For this review, take the finished solid that the model builds, in its own axes (mm). Face numbers are marked on the shaded views. A direction names the side the tool comes from. Give positions to 0.01 mm unless a question says otherwise; leave off trailing zeros. Loops run counter-clockwise (first coordinate to the right, second up) from the corner with the lowest first, then second, coordinate; pieces in that order, holes last. Notation, with made-up numbers: (26.25, -29) - (38.25, -29) arc R25 ccw to (38.25, -15) - close; hole circle Ø11 at (49.5, 51.25). An arc over 180 degrees is marked (long way). Answer in a Markdown table with one row per item.
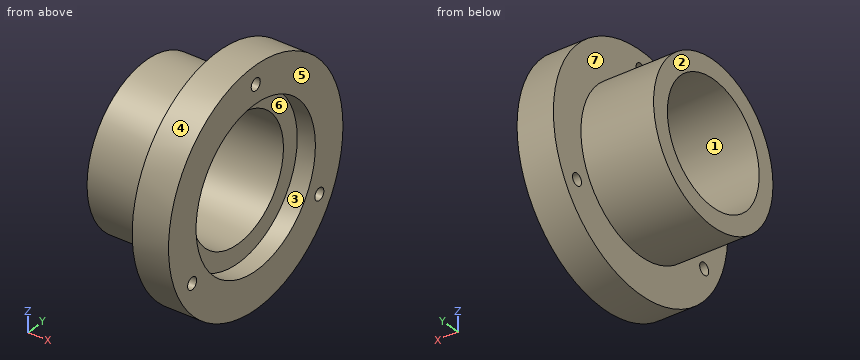
```python
from build123d import *

# Parameters (mm, degrees)
F0_R        = 24.13
F1_DEPTH    = 22.86
F2_R        = 16.51
F3_DEPTH    = 3.81
F4_R        = 12.7
F5_DEPTH    = 19.05
F6_R        = 24.13
F6_R_2      = 16.51
F7_DEPTH    = 15.24
F8_R        = 1.25
F7_FACE_R   = 24.13
F7_FACE_R_2 = 16.51
F9_DEPTH    = 25.4


with BuildPart() as f1:
    # F0 (on Right) → F1 (new body)
    with BuildSketch(Plane.YZ):
        Circle(F0_R)
    extrude(amount=F1_DEPTH)

    # F2 (on face) → F3 (cut)
    with BuildSketch(Plane.YZ.offset(22.86)):
        Circle(F2_R)
    extrude(amount=-F3_DEPTH, mode=Mode.SUBTRACT)

    # F4 (on face) → F5 (cut, through all)
    with BuildSketch(Plane.YZ.offset(19.05)):
        Circle(F4_R)
    extrude(amount=-F5_DEPTH, mode=Mode.SUBTRACT)

    # F6 (on face) → F7 (cut)
    with BuildSketch(Plane(origin=(0, 0, 0), x_dir=(0, -1, 0), z_dir=(-1, 0, 0))):
        Circle(F6_R)
        Circle(F6_R_2, mode=Mode.SUBTRACT)
    extrude(amount=-F7_DEPTH, mode=Mode.SUBTRACT)

    # F8 (on face) + F7_face (on face) → F9 (cut)
    with BuildSketch(Plane.YZ.offset(22.86)):
        with Locations((0, 20.32)):
            Circle(F8_R)
        with Locations((-17.5976362049, -10.16)):
            Circle(F8_R)
        with Locations((17.5976362049, -10.16)):
            Circle(F8_R)
    with BuildSketch(Plane(origin=(15.24, 0, 0), x_dir=(0, -1, 0), z_dir=(-1, 0, 0))):
        Circle(F7_FACE_R)
        Circle(F7_FACE_R_2, mode=Mode.SUBTRACT)
    extrude(amount=-F9_DEPTH, dir=(1, 0, 0), mode=Mode.SUBTRACT)


solid = f1.part
```
1. Clearance check with flat-ended pins moving along their axes: pin 1 (3 mm diameter, centred on y = 17.6, z = -10.16, fed in from -X); pin 2 (2 mm diameter, centred on x = 6.5, y = -11, fed in from +Z); pin 3 (16.5 mm diameter, centred on y = 1.5, z = -1.5, fed in from +X); pin 4 (2 mm diameter, centred on x = 16, y = -15.5, fed in from -Z). State where each tip first meets the part, or that it passes through.
Values:
| item | result |
|---|---|
| pin 1 | stops at x = 15.24 |
| pin 2 | stops at z = 13.14 |
| pin 3 | passes through |
| pin 4 | stops at z = -19.29 |
2. For the marked faces 5, 6 and 7, list the 3-axis set-ups (+Z, -Z, +X, -X, +Y, -Y) from which the entire face can be reached by the end or side of a thin tool; tool diameter is ignored.
Values:
| item | result |
|---|---|
| face 5 | +Z, -Z, +X, +Y, -Y |
| face 6 | +X |
| face 7 | -X |
3. We need section D-D, the plane z = -10.16. Give the boundary of the cut face in (x, y), and give its area (3 significant figures).
Values:
| item | result |
|---|---|
| outline | (0, -13.01) - (15.24, -13.01) - (15.24, -16.35) - (22.86, -16.35) - (22.86, -13.01) - (19.05, -13.01) - (19.05, -7.62) - (0, -7.62) - close; (0, 7.62) - (19.05, 7.62) - (19.05, 13.01) - (22.86, 13.01) - (22.86, 16.35) - (15.24, 16.35) - (15.24, 13.01) - (0, 13.01) - close; (15.24, -21.89) - (22.86, -21.89) - (22.86, -18.85) - (15.24, -18.85) - close; (15.24, 18.85) - (22.86, 18.85) - (22.86, 21.89) - (15.24, 21.89) - close |
| area | 303 mm^2 |
4. We need section B-B, the plane z = 20.32. Give the boundary of the cut face in (x, y).
Values:
| item | result |
|---|---|
| outline | (15.24, -13.01) - (22.86, -13.01) - (22.86, -1.25) - (15.24, -1.25) - close; (15.24, 1.25) - (22.86, 1.25) - (22.86, 13.01) - (15.24, 13.01) - close |
5. We need section A-A, the plane y = 0. Give the boundary of the cut face in (x, z).
Values:
| item | result |
|---|---|
| outline | (0, -16.51) - (15.24, -16.51) - (15.24, -24.13) - (22.86, -24.13) - (22.86, -16.51) - (19.05, -16.51) - (19.05, -12.7) - (0, -12.7) - close; (0, 12.7) - (19.05, 12.7) - (19.05, 16.51) - (22.86, 16.51) - (22.86, 19.07) - (15.24, 19.07) - (15.24, 16.51) - (0, 16.51) - close; (15.24, 21.57) - (22.86, 21.57) - (22.86, 24.13) - (15.24, 24.13) - close |
6. We need section C-C, the plane x = 1.5. Give the boundary of the cut face in (y, z), and give its area (3 significant figures).
Values:
| item | result |
|---|---|
| outline | circle Ø33.02 at (0, 0); hole circle Ø25.4 at (0, 0) |
| area | 350 mm^2 |
7. Wall thickness on line 1 (Z direction, x = 20.3, y = 0); line 2 (Y direction, x = 10.5, z = -0.5); line 3 (Z direction, x = 4.5, y = 0): over which ranges is each line inside the solid? List them lowest first. Write a range as [from, to].
Values:
| item | result |
|---|---|
| line 1 | z = [-24.13, -16.51], [16.51, 19.07], [21.57, 24.13] |
| line 2 | y = [-16.5, -12.69], [12.69, 16.5] |
| line 3 | z = [-16.51, -12.7], [12.7, 16.51] |
8. Mouldability with a two-part tool opening along Z and no side actions: class the marked faces 1, 2, 3 and 4 as released by +Z, released by -Z, zero draft, split by the parting line, or undercut.
Values:
| item | result |
|---|---|
| face 1 | undercut |
| face 2 | zero draft |
| face 3 | undercut |
| face 4 | split by the parting line |
